```python
from build123d import *

# Parameters (mm, degrees)
F0_R     = 10
F1_DEPTH = 25
F2_W     = 8
F2_H     = 8
F3_DEPTH = 50.001
F7_R     = 7.5
F8_DEPTH = 20


with BuildPart() as f1:
    # F0 (on Top) → F1 (new body, symmetric)
    with BuildSketch(Plane.XY):
        Circle(F0_R)
    extrude(amount=F1_DEPTH, both=True)

    # F2 (on face) → F3 (cut, through all)
    with BuildSketch(Plane.XY.offset(25)):
        Rectangle(F2_W, F2_H)
    extrude(amount=-F3_DEPTH, mode=Mode.SUBTRACT)

    # F4 (on Front) → F6 (revolve, cut)
    with BuildSketch(Plane.XZ):
        Polygon((-10, 10), (-10, 0), (-7, 5), align=None)
    revolve(axis=Axis((0, 0, 10.121179), (0, 0, 1)), mode=Mode.SUBTRACT)

    # F7 (on face) → F8 (cut)
    with BuildSketch(Plane(origin=(0, 0, -25), x_dir=(1, 0, 0), z_dir=(0, 0, -1))):
        Circle(F7_R)
    extrude(amount=-F8_DEPTH, mode=Mode.SUBTRACT)


solid = f1.part
```
Verification items for the finished model (mm, model axes). A direction names the side the tool comes from. Give positions to 0.01 mm unless a question says otherwise; leave off trailing zeros. Order: outer loops, then holes, each group sorted by start corner. A loop starts at its lowest first (then second) coordinate and runs counter-clockwise, first axis right, second up. Notation, with made-up numbers: (-40, 72.5) -> (8, 72.5) arc R30 ccw to (8, 108.5) -> close; hole circle Ø8 at (67.5, 29.5). An arc over 180 degrees is marked (long way). One line per item, written item: value.
(1) Sectioned sample at C-C on z = 3. Record the cut outline in (x, y).
Final values:
outline: circle Ø16.4 at (0, 0); hole (-4, -4) -> (4, -4) -> (4, 4) -> (-4, 4) -> close
(2) Tool access check on faces 1 (the face through (0, -4, 10)), 2 (the face through (5.671, 4.348, 4.757)), 3 (the face through (0, 5, -5)), 4 (the face through (-0.1, -4.3, 25)). Record the directions out of +Z, -Z, +X, -X, +Y, -Y that give a thin tool (end or side, any length) a straight path to the whole face; none if there is none.
Final values:
face 1: +Z, -Z
face 2: none
face 3: -Z
face 4: +Z, +X, -X, +Y, -Y
(3) Sectioned sample at D-D on z = 19. Record the cut outline in (x, y), then the cut area to 3 significant figures.
Final values:
outline: circle Ø20 at (0, 0); hole (-4, -4) -> (4, -4) -> (4, 4) -> (-4, 4) -> close
area: 250 mm^2
(4) Scan lines: line 1 along Y through (x, z) = (0, -18); line 2 along Y through (x, z) = (0, 17). Record each from-to range of solid material in increasing order. Write a range as [from, to].
Final values:
line 1: [-10, -7.5], [7.5, 10]
line 2: [-10, -4], [4, 10]
(5) Draft check along Y on faces 5 (the face through (0, 4, 10)), 6 (the face through (-6.856, -2.159, 5.313)), 7 (the face through (4, 7, -25)). Enter one of: pulls with the +Y half, pulls with the -Y half, needs draft (parallel to the pull), parting line crosses it, or undercut.
Final values:
face 5: undercut
face 6: parting line crosses it
face 7: needs draft
(6) Gauge pin test, flat ends, axial feed: pin 1 (2.5 mm diameter, centred on x = -1.5, z = 9, fed in from +Y); pin 2 (4 mm diameter, centred on y = -7, z = 16.5, fed in from -X); pin 3 (1.5 mm diameter, centred on y = 2, z = -18, fed in from -X). Record the tip position at first contact, or that the pin passes through.
Final values:
pin 1: y = 9.97
pin 2: x = -8.66
pin 3: x = -9.92
(7) Sectioned sample at A-A on y = 0. Record the cut outline in (x, z).
Final values:
outline: (-10, -25) -> (-7.5, -25) -> (-7.5, -5) -> (-4, -5) -> (-4, 25) -> (-10, 25) -> (-10, 10) -> (-7, 5) -> (-10, 0) -> close; (4, -5) -> (7.5, -5) -> (7.5, -25) -> (10, -25) -> (10, 0) -> (7, 5) -> (10, 10) -> (10, 25) -> (4, 25) -> close
